Check sheet for the drawn part. Datum: minimum x, y, z corner. Units: mm. Give positions to 0.01 mm unless a question says otherwise; leave off trailing zeros. Order: outer loops, then holes, each group sorted by start corner. A loop starts at its lowest first (then second) coordinate and runs counter-clockwise, first axis right, second up. Notation, with made-up numbers: (83, 6) -> (102, 6) arc R11 cw to (102, 25) -> close; hole circle Ø2 at (-23, 0). An arc over 180 degrees is marked (long way). Return JSON: item names as keys, results as strings. Group by question number.
(1) Cross-section at B-B on z = 3.3. State how many separate pieces and enclosed holes the cut face has, then the cut area to 3 significant figures.
(2) Cross-section at A-A on y = 12.5. Enter the section's corners in (x, z), then the cut area to 3 significant figures.
(3) Cross-section at D-D on y = 27. Enter the section's corners in (x, z).
(4) Thickness scan on line 1 along X through (y, z) = (11, 4.6); line 2 along Y through (x, z) = (41, 3.95); line 3 along Y through (x, z) = (10, 3.9). Record the ranges inside material, lowest first.
(5) Cross-section at C-C on x = 37.5. Enter the section's corners in (y, z).
(6) Release check for a two-part mould opening along Y. For the marked faces 1, 2 and 3 record: pulls with the +Y half, pulls with the -Y half, needs draft (parallel to the pull), parting line crosses it, or undercut.
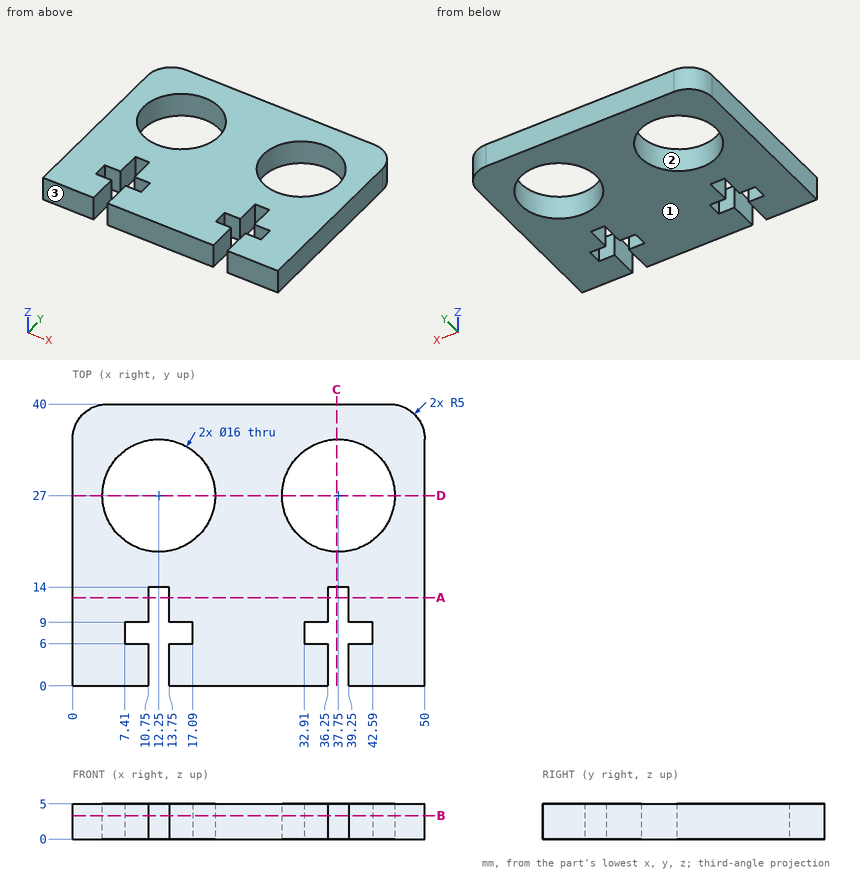
Verdict:
{
 "1": {"separate pieces": "1", "enclosed holes": "2", "area": "1,460 mm²"},
 "2": {"outline": "(0, 0) -> (10.75, 0) -> (10.75, 5) -> (0, 5) -> close; (13.75, 0) -> (36.25, 0) -> (36.25, 5) -> (13.75, 5) -> close; (39.25, 0) -> (50, 0) -> (50, 5) -> (39.25, 5) -> close", "area": "220 mm²"},
 "3": {"outline": "(0, 0) -> (4.25, 0) -> (4.25, 5) -> (0, 5) -> close; (20.25, 0) -> (29.75, 0) -> (29.75, 5) -> (20.25, 5) -> close; (45.75, 0) -> (50, 0) -> (50, 5) -> (45.75, 5) -> close"},
 "4": {"line 1": "0 to 10.75, 13.75 to 36.25, 39.25 to 50", "line 2": "0 to 6, 9 to 19.69, 34.31 to 40", "line 3": "0 to 6, 9 to 19.32, 34.68 to 40"},
 "5": {"outline": "(14, 0) -> (19, 0) -> (19, 5) -> (14, 5) -> close; (35, 0) -> (40, 0) -> (40, 5) -> (35, 5) -> close"},
 "6": {"face 1": "needs draft", "face 2": "undercut", "face 3": "pulls with the -Y half"}
}
